```python
from build123d import *

# Parameters (mm, degrees)
F0_W     = 127
F0_H     = 127
F1_DEPTH = 127
F2_R     = 38.1
F3_DEPTH = 127.001
F4_R     = 5.08


with BuildPart() as f1:
    # F0 (on Front) → F1 (new body)
    with BuildSketch(Plane.XZ):
        with Locations((-2e-06, -21.783345)):
            Rectangle(F0_W, F0_H)
    extrude(amount=F1_DEPTH)

    # F2 (on face) → F3 (cut, through all)
    with BuildSketch(Plane(origin=(0, 0, -85.283345), x_dir=(1, 0, 0), z_dir=(0, 0, -1))):
        with Locations((-2e-06, 63.5)):
            Circle(F2_R)
    extrude(amount=-F3_DEPTH, mode=Mode.SUBTRACT)

    # F4
    f4_edges = [f1.edges().sort_by_distance(p)[0] for p in [
        (-38.100002, -63.5, -85.283345),
        (38.099998, -63.5, -21.783345),
        (-38.100002, -63.5, 41.716655),
        (-2e-06, 0, -85.283345),
    ]]
    fillet(f4_edges, radius=F4_R)


solid = f1.part
```
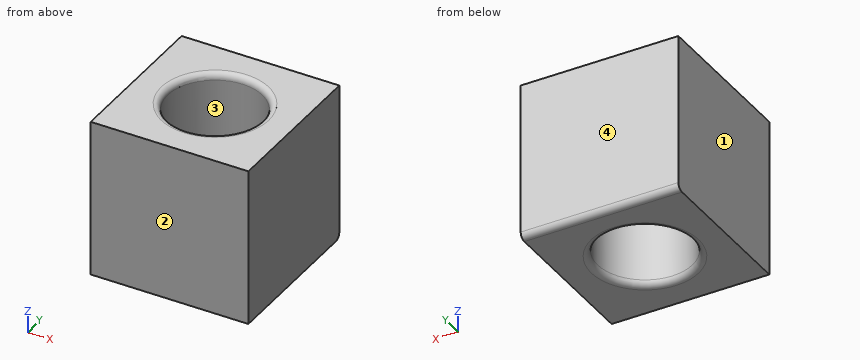
The model under review builds one solid part; all positions refer to its coordinate system, in mm. Face numbers are marked on the shaded views. Round coordinates to 2 decimals unless told otherwise and drop trailing zeros. Order: outer loops, then holes, each group sorted by start corner. A loop starts at its lowest first (then second) coordinate and runs counter-clockwise, first axis right, second up. Notation, with made-up numbers: M -10,51.5 L 45,51.5 A23 ccw 45,62.5 Z; hole C -16,-9 d10. An arc over 180 degrees is marked long. Use a Markdown table: item, result.
1) Insertion check: pin 1 (1 mm diameter, centred on x = 37.5, y = -54, fed in from -Z). The pin has a flat end and moves straight along its axis. Give the tip position at first contact, or say it passes through.
Report:
| item | result |
|---|---|
| pin 1 | z = -83.34 |
2) Consider section B-B (z = 5.5). Write out the cut boundary in (x, y).
Report:
| item | result |
|---|---|
| outline | M -63.5,-127 L 63.5,-127 L 63.5,0 L -63.5,0 Z; hole C 0,-63.5 d76.2 |
3) Consider section A-A (y = -63.5). Write out the cut boundary in (x, z).
Report:
| item | result |
|---|---|
| outline | M -63.5,-85.28 L -43.18,-85.28 A5.08 ccw -38.1,-80.2 L -38.1,36.64 A5.08 ccw -43.18,41.72 L -63.5,41.72 Z; M 38.1,-80.2 A5.08 ccw 43.18,-85.28 L 63.5,-85.28 L 63.5,41.72 L 43.18,41.72 A5.08 ccw 38.1,36.64 Z |
4) Draft analysis for pull direction Y (two halves, no side actions). For the marked faces 1, 2, 3 and 4, state which applies: released by +Y, released by -Y, zero draft, split by the parting line, or undercut.
Report:
| item | result |
|---|---|
| face 1 | zero draft |
| face 2 | released by -Y |
| face 3 | undercut |
| face 4 | released by +Y |
5) Wall thickness on line 1 along Y through (x, z) = (0.5, -49); line 2 along X through (y, z) = (-63.5, 12); line 3 along Z through (x, y) = (38, -43.5): over which ranges is each line inside the solid? List them lowest first. Write a range as [from, to].
Report:
| item | result |
|---|---|
| line 1 | [-127, -101.6], [-25.4, 0] |
| line 2 | [-63.5, -38.1], [38.1, 63.5] |
| line 3 | [-85.28, 41.71] |
